Model file for the job. Use its own axes, mm. A direction names the side the tool comes from. Give positions to 0.01 mm unless a question says otherwise; leave off trailing zeros. Order: outer loops, then holes, each group sorted by start corner. A loop starts at its lowest first (then second) coordinate and runs counter-clockwise, first axis right, second up. Notation, with made-up numbers: (15, 40.5) - (40, 40.5) arc R31 ccw to (40, 66.5) - close; hole circle Ø8 at (-32.75, 30.25). An arc over 180 degrees is marked (long way). Return JSON: item names as keys, results as strings. Group by question number.
Autodesk Inventor part; units mm, degrees
ref_plane "Work Plane1" through (29, 0, 0) normal (0, -1, 0) x (1, 0, 0)
ref_plane "YZ Plane" through (0, 0, 0) normal (1, 0, 0) x (0, 1, 0)
ref_plane "XZ Plane" through (0, 0, 0) normal (0, 1, 0) x (-1, 0, 0)
sketch "Sketch1" plane through (0, 0, 0) normal (0, 0, 1) x (1, 0, 0)
  line L0 (-0.8667, 0) -> (35, 0)
  line L1 (35, 0) -> (35, 1.5)
  line L2 (35, 1.5) -> (28.25, 1.5)
  line L3 (28.25, 1.5) -> (27.9432, 1.5)
  line L4 (27.9432, 1.5) -> (0, 1.5)
  line L5 (0, 1.5) -> (0, 2.75)
  line L6 (0, 2.75) -> (-3, 2.75)
  line L7 (-3, 2.75) -> (-3, 1.4434)
  line L8 (-3, 1.4434) -> (-1.7, 1.4434)
  line L9 (-1.7, 1.4434) -> (-0.8667, 0)
  line L10 (-10.6, 0) -> (42.6, 0)
  line L11 (0, -0.55) -> (0, 3.3)
  line L12 (28.25, 1.5) -> (0, 1.5) construction
  dimension "d1" = 6.75
  dimension "d2" = 0.3068
  dimension "d3" = 3
  dimension "d4" = 1.3
  dimension "d5" = 60
  dimension "d6" = 3
  dimension "d7" = 3
  dimension "d8" = 2.8868
  dimension "d9" = 5.5
  dimension "d26" = 35
revolve "Body" add sketch "Sketch1" angle 360 about axis through (-0.8667, 0, 0) along (1, 0, 0)
sketch "Sketch2" plane through (-3, 0, 0) normal (-1, 0, 0) x (0, 0, 1)
  circle A0 centre (0, 0) radius 1.4434
  line L0 (0, -3.85) -> (0, 3.85)
  line L1 (-3.85, 0) -> (3.85, 0)
  line L2 (1.4434, 0) -> (0.7217, -1.25)
  line L3 (0.7217, -1.25) -> (-0.7217, -1.25)
  line L4 (-0.7217, -1.25) -> (-1.4434, 0)
  line L5 (-1.4434, 0) -> (-0.7217, 1.25)
  line L6 (-0.7217, 1.25) -> (0.7217, 1.25)
  line L7 (0.7217, 1.25) -> (1.4434, 0)
extrude "Slot" add sketch "Sketch2" against normal up to next contours L7 A0 | A0 L2 | L6 L0 A0 | A0 L0 L3 | L0 L6 A0 | A0 L3 L0 | L4 A0 | A0 L5
fillet "Fillet1" radius 0.3 1 edges at (-3, -2.75, 0)
thread "Thread"
chamfer "Chamfer1" distance 0.3067 distance2 0.3067 1 edges at (35, -1.5, 0) measured on face at (35, -0.8773, -0.3972)
ref_plane "Work Plane1" through (29, 0, 0) normal (0, -1, 0) x (1, 0, 0)
fillet "Fillet2" radius 0.1 1 edges at (0, -1.5, 0)
equation "\"d1\" = GEL"
equation "\"d3\" = KOH"
equation "\"d4\" = INTI"
equation "\"d6\" = GD"
equation "\"d7\" = BDM"
equation "\"d8\" = 1.1547 * SW"
equation "\"d9\" = KOD"
equation "\"d30\" = R"
equation "\"d17\" = RR"
equation "\"d13\" = GEL"
equation "\"d15\" = -0.5 * SPD + 0.5 * GD"
equation "\"d16\" = GUL"
equation "\"GD\" = NND"
equation "\"NLG\" = 8"
equation "\"GEL\" = 6.75"
equation "\"KOD\" = 5.5"
equation "\"KOH\" = NND"
equation "\"INTI\" = 1.3"
equation "\"GAL\" = 0.61345 * PTC"
equation "\"GUL\" = 0.61345 * PTC"
equation "\"BDM\" = NND"
equation "\"SW\" = 2.5"
equation "\"RR\" = 0.1 * NND"
equation "\"SPD\" = NND - 1.2269 * PTC"
equation "\"R\" = 0.1"
equation "\"PHH\" = 0.13"
equation "\"GD1\" = THREADDIA - 1.2269 * PTC"
equation "\"THREADDIA\" = 3"
equation "\"FAWI\" = 45deg"
equation "\"PTC\" = 0.5"
equation "\"KOH1\" = 2.7"
equation "\"NND\" = 3"
equation "\"TOA\" = 30deg"
equation "\"E0\" = 1.155 * SW"
properties part number "AS 1420 - 1973 - M3 x 8" material "Steel, Mild"
(1) Pull direction Y, two halves, no side cores. Call faces 1 (the face through (-2, -1.25, 0)), 2 (the face through (-3, -1.1, 1.1)), 3 (the face through (17.15, -1.5, -0.07)): released by +Y, released by -Y, zero draft, split by the parting line, or undercut.
(2) 3-axis set-ups, long thin cutter, end or side, ignore diameter. For faces 4 (the face through (0, 2, 0)), 5 (the face through (-2.3, -0.63, -1.08)), 6 (the face through (35, 0, 0)): which of +Z, -Z, +X, -X, +Y, -Y reach the whole face in a straight line?
(3) Drop flat-ended pins along their axis: pin 1 Ø2 at (x, y) = (2, -1) entering from -Z; pin 2 Ø2 at (x, y) = (22.5, -1.5) entering from +Z; pin 3 Ø1 at (y, z) = (1, -2) entering from +X. Give the stop position or say it passes through.
(4) Drill centre lines: L1, parallel to X at y = -1.4, z = -1.5; L2, parallel to Z at x = 20.5, y = 0.9; L3, parallel to X at y = -0.7, z = 0.55. Where is each one in solid material? Low to high.
(5) Slice it at A-A (x = 31.5). Give the cut face in (y, z), and give its area (3 significant figures).
Result set:
{
 "1": {"face 1": "undercut", "face 2": "zero draft", "face 3": "split by the parting line"},
 "2": {"face 4": "+X", "face 5": "-X", "face 6": "+Z, -Z, +X, +Y, -Y"},
 "3": {"pin 1": "stops at z = -1.5", "pin 2": "stops at z = 1.41", "pin 3": "stops at x = 0"},
 "4": {"L1": "x = -3 to 0", "L2": "z = -1.2 to 1.2", "L3": "x = -1.38 to 35"},
 "5": {"outline": "circle Ø3 at (0, 0)", "area": "7.07 mm²"}
}
